```python
from build123d import *

# Parameters (mm, degrees)
F1_DEPTH = 8
F2_R     = 3
F4_D     = 4.4
F6_D     = 4.4


with BuildPart() as f1:
    # F0 (on Top) → F1 (new body)
    with BuildSketch(Plane.XY):
        Polygon((0, 30), (0, 0), (0, -30), (5, -30), (5, -7.4492068961), (19.0707250684, -7.4492068961), (19.0707250684, -30), (24.0707250684, -30), (24.0707250684, 30), align=None)
    extrude(amount=F1_DEPTH)

    # F2
    f2_edges = [f1.edges().sort_by_distance(p)[0] for p in [
        (21.570725, -30, 8),
        (2.5, -30, 8),
        (12.035363, 30, 8),
    ]]
    fillet(f2_edges, radius=F2_R)

    # F4 (through all)
    with Locations(Plane.YZ.offset(24.0707250684)):
        with Locations((-27, 5)):
            Hole(F4_D / 2)

    # F6 (through all)
    with Locations(Plane.YZ.offset(24.0707250684)):
        with Locations((0, 3.8463051897)):
            Hole(F6_D / 2)


solid = f1.part
```
For this review, take the finished solid that the model builds, in its own axes (mm). A direction names the side the tool comes from. Round coordinates to 2 decimals unless told otherwise and drop trailing zeros. Write each loop counter-clockwise with the first axis right and the second up, starting at its lowest first coordinate (ties: lowest second). Pieces come first, ordered by that corner, then holes. Notation, with made-up numbers: (67, 49.25) - (89, 49.25) arc R33 cw to (89, 85.25) - close; hole circle Ø4 at (-16, 71). An arc over 180 degrees is marked (long way). Answer as CSV lines item,"result". Start each with the question number.
(1) Add section D-D, the plane x = 18. State the section outline as (y, z) points, plus the area to 3 significant figures.
(2) Add section C-C, the plane y = 0. State the section outline as (x, z) points, plus the area to 3 significant figures.
(3) Mouldability with a two-part tool opening along Z and no side actions: class faces 3 (the flat face through (12, 7, 0)), 4 (the flat face through (5, -19, 4)), 5 (the cylindrical face through (21.61, -29.14, 7.1)), 6 (the cylindrical face through (21.536, -24.802, 5.097)) as +Z half, -Z half, draft (parallel to the pull), parting line (faces both ways), or undercut.
(4) For pin 1 (2.5 mm diameter, centred on y = 0, z = 3.85, fed in from -X); pin 2 (4 mm diameter, centred on x = 14, z = 2, fed in from -Y), all flat-tipped, find the tip position at first contact; note any pin that passes through.
(5) For line 1 (Z direction, x = 20.6, y = -27); line 2 (X direction, y = -7.5, z = 4.75); line 3 (Z direction, x = 11.5, y = 0), list the stretches that pass through material, from the lowest coordinate up.
(6) Add section B-B, the plane x = 2.5. State the section outline as (y, z) points.
(7) Machinability: for faces 1 (the flat face through (12, -7.449, 4)), 2 (the cylindrical face through (2.54, -29.14, 7.1)), which of the approach directions +Z, -Z, +X, -X, +Y, -Y give a long, thin tool a straight path to every point of the face, cutting with its end or side? Answer none if there is none.
(8) Add section A-A, the plane y = -19. State the section outline as (x, z) points, plus the area to 3 significant figures.
From the geometry:
1,outline,"(-7.45, 0) - (30, 0) - (30, 5) arc R3 ccw to (27, 8) - (-7.45, 8) - close; hole circle Ø4.4 at (0, 3.85)"
1,area,"282 mm²"
2,outline,"(0, 0) - (24.07, 0) - (24.07, 1.65) - (0, 1.65) - close; (0, 6.05) - (24.07, 6.05) - (24.07, 8) - (0, 8) - close"
2,area,"86.7 mm²"
3,face 3,"-Z half"
3,face 4,"draft"
3,face 5,"+Z half"
3,face 6,"undercut"
4,pin 1,"passes through"
4,pin 2,"stops at y = -7.45"
5,line 1,"z = 0 to 2.8, 7.2 to 8"
5,line 2,"x = 0 to 5, 19.07 to 24.07"
5,line 3,"z = 0 to 1.65, 6.05 to 8"
6,outline,"(-30, 0) - (30, 0) - (30, 5) arc R3 ccw to (27, 8) - (-27, 8) arc R3 ccw to (-30, 5) - close; hole circle Ø4.4 at (-27, 5); hole circle Ø4.4 at (0, 3.85)"
7,face 1,"+Z, -Z, -Y"
7,face 2,"+Z, +X, -X, -Y"
8,outline,"(0, 0) - (5, 0) - (5, 8) - (0, 8) - close; (19.07, 0) - (24.07, 0) - (24.07, 8) - (19.07, 8) - close"
8,area,"80.0 mm²"
